from build123d import *

# Parameters (mm, degrees)
EXTRUDE_1_DEPTH          = 12
CHAMFER_1_SIZE           = 3
SKETCH_2_R               = 3.25
CUT_EXTRUDE_1_DEPTH      = 13
PATTERN_CIRCULAR_1_COUNT = 6
SKETCH_4_R               = 4
CUT_EXTRUDE_2_DEPTH      = 13
PATTERN_CIRCULAR_2_COUNT = 6
SKETCH_5_R               = 4.5
CUT_EXTRUDE_3_DEPTH      = 13
SKETCH_9_R               = 4.5
CUT_EXTRUDE_5_DEPTH      = 13
PATTERN_CIRCULAR_3_COUNT = 6


with BuildPart() as part:
    # 草圖1 → 填料-伸長1 (new body)
    with BuildSketch(Plane(origin=(0, 0, 0), x_dir=(1, 0, 0), z_dir=(0, 1, 0))):
        Polygon((75, 43.301270189), (0, 86.602540378), (-75, 43.301270189), (-75, -43.301270189), (0, -86.602540378), (75, -43.301270189), align=None)
    extrude(amount=EXTRUDE_1_DEPTH)

    # 導角1
    chamfer_1_edges = [part.edges().sort_by_distance(p)[0] for p in [
        (-37.5, 12, -64.951905284),
        (-75, 12, 0),
        (-37.5, 12, 64.951905284),
        (37.5, 12, 64.951905284),
        (75, 12, 0),
        (37.5, 12, -64.951905284),
    ]]
    chamfer(chamfer_1_edges, length=CHAMFER_1_SIZE)

    # 草圖2 → 除料-伸長1 (cut, through all)
    with BuildSketch(Plane.XZ):
        with Locations((65, -37.5)):
            Circle(SKETCH_2_R)
    cut_extrude_1 = extrude(amount=-CUT_EXTRUDE_1_DEPTH, mode=Mode.SUBTRACT)

    # 環狀複製排列1: 除料-伸長1 ×6 about axis
    pattern_circular_1_axis = Axis((0, 0, 0), (0, 1, 0))
    for i in range(1, PATTERN_CIRCULAR_1_COUNT):
        add(cut_extrude_1.rotate(pattern_circular_1_axis, i * 360 / PATTERN_CIRCULAR_1_COUNT), mode=Mode.SUBTRACT)

    # 草圖4 → 除料-伸長2 (cut, through all)
    with BuildSketch(Plane.XZ):
        with Locations((65, 0)):
            Circle(SKETCH_4_R)
    cut_extrude_2 = extrude(amount=-CUT_EXTRUDE_2_DEPTH, mode=Mode.SUBTRACT)

    # 環狀複製排列2: 除料-伸長2 ×6 about axis
    pattern_circular_2_axis = Axis((0, 0, 0), (0, 1, 0))
    for i in range(1, PATTERN_CIRCULAR_2_COUNT):
        add(cut_extrude_2.rotate(pattern_circular_2_axis, i * 360 / PATTERN_CIRCULAR_2_COUNT), mode=Mode.SUBTRACT)

    # 草圖5 → 除料-伸長3 (cut, through all)
    with BuildSketch(Plane.XZ):
        Circle(SKETCH_5_R)
    extrude(amount=-CUT_EXTRUDE_3_DEPTH, mode=Mode.SUBTRACT)

    # 草圖9 → 除料-伸長5 (cut, through all)
    with BuildSketch(Plane.XZ):
        with Locations((0, 23.006385047)):
            Circle(SKETCH_9_R)
        with Locations((9.960213319, 17.257980865)):
            Circle(SKETCH_9_R)
        with Locations((19.920426639, 11.509576684)):
            Circle(SKETCH_9_R)
        with Locations((34.644220241, 20.016655103)):
            Circle(SKETCH_9_R)
        with Locations((50.23411935, 29.024149899)):
            Circle(SKETCH_9_R)
        with Locations((25.117059675, 43.52012566)):
            Circle(SKETCH_9_R)
        with Locations((17.326919147, 30.011104301)):
            Circle(SKETCH_9_R)
        with Locations((0, 40.011104429)):
            Circle(SKETCH_9_R)
        with Locations((0, 58.016101422)):
            Circle(SKETCH_9_R)
    cut_extrude_5 = extrude(amount=-CUT_EXTRUDE_5_DEPTH, mode=Mode.SUBTRACT)

    # 環狀複製排列3: 除料-伸長5 ×6 about axis
    pattern_circular_3_axis = Axis((0, 0, 0), (0, 1, 0))
    for i in range(1, PATTERN_CIRCULAR_3_COUNT):
        add(cut_extrude_5.rotate(pattern_circular_3_axis, i * 360 / PATTERN_CIRCULAR_3_COUNT), mode=Mode.SUBTRACT)


solid = part.part
Part model, mm, in its own coordinate system. Give positions to 0.01 mm unless a question says otherwise; leave off trailing zeros. Order: outer loops, then holes, each group sorted by start corner. A loop starts at its lowest first (then second) coordinate and runs counter-clockwise, first axis right, second up. Notation, with made-up numbers: (37.5, 81) -> (81.5, 81) arc R10 cw to (81.5, 85) -> close; hole circle Ø6 at (81, 1.5). An arc over 180 degrees is marked (long way). Use one line per item in the form item = value.
(1) Saw through at A-A (z = 56). Write the cut outline in (x, y).
Solution:
outline = (-53.01, 0) -> (-36.49, 0) -> (-36.49, 12) -> (-47.01, 12) -> (-53.01, 9) -> close; (-28.51, 0) -> (-4.04, 0) -> (-4.04, 12) -> (-28.51, 12) -> close; (4.02, 0) -> (28.51, 0) -> (28.51, 12) -> (4.02, 12) -> close; (36.49, 0) -> (53.01, 0) -> (53.01, 9) -> (47.01, 12) -> (36.49, 12) -> close
(2) Saw through at B-B (z = 0). Count the separate pieces of the cut face and the enclosed holes in it, then the cut area to 3 significant figures.
Solution:
separate_pieces = 10
enclosed_holes = 0
area = 843 mm²
(3) Pull direction Z, two halves, no side cores. Call faces 1 (the face through (37.265, 10.521, -63.332)), 2 (the face through (-4.51, 5.92, 40.11)), 3 (the face through (-75, 4, -1)): +Z half, -Z half, draft (parallel to the pull), parting line (faces both ways), or undercut.
Solution:
face_1 = -Z half
face_2 = undercut
face_3 = draft
(4) Flat gauge pins, fed straight in: P1, Ø5, axis at y = 5.5, z = 67, coming from the -X side; P2, Ø6, axis at y = 2, z = -48, coming from the -X side; P3, Ø1, axis at x = -24, y = 9, coming from the -Z side. Where does each tip first touch, or does it go through?
Solution:
P1 = -38.28
P2 = -72.06
P3 = -73.03
(5) Saw through at D-D (x = -43.5). Write the cut outline in (y, z).
Solution:
outline = (0, -61.49) -> (9, -61.49) -> (12, -58.02) -> (12, 58.02) -> (9, 61.49) -> (0, 61.49) -> close
(6) Drill centre lines: line 1 (X direction, y = 1, z = 40.5); line 2 (X direction, y = 6.5, z = -25); line 3 (Z direction, x = 65, y = 6). Where is each one in solid material? Low to high. Write a range as from..to.
Solution:
line_1 = -75..-66.25, -63.75..-28.47, -21.79..-4.49, 4.47..21.78, 28.45..63.63, 66.32..75
line_2 = -75..-52.29, -48.2..-4.03, 4.04..48.18, 52.33..75
line_3 = -49.07..-40.75, -34.25..-4, 4..34.29, 40.79..49.07
